Verification items for the finished model (mm, model axes). Face numbers are marked on the shaded views. A direction names the side the tool comes from. Give positions to 0.01 mm unless a question says otherwise; leave off trailing zeros. Loops run counter-clockwise (first coordinate to the right, second up) from the corner with the lowest first, then second, coordinate; pieces in that order, holes last. Notation, with made-up numbers: M 12.5,-21 L 24.5,-21 A22 ccw 24.5,-12 Z; hole C -23.75,-30 d6. An arc over 180 degrees is marked long. Use CSV: the item, a comma, the result in double quotes.
from build123d import *

# Parameters (mm, degrees)
EXTRUDE_1_DEPTH     = 29
EXTRUDE_2_DEPTH     = 5
CHAMFER_1_SIZE      = 1
SKETCH_4_W          = 2
SKETCH_4_H          = 3.10400654
SKETCH_4_H_2        = 3.326169865
CUT_EXTRUDE_1_DEPTH = 30


with BuildPart() as part:
    # 草图1 → 凸台-拉伸1 (new body)
    with BuildSketch(Plane.XY):
        Polygon((-19.832016219, -9.875726629), (-3.832016219, -9.875726629), (-8.832016219, -4.875726629), (-14.832016219, -4.875726629), align=None)
    extrude(amount=EXTRUDE_1_DEPTH)

    # 草图3 → 凸台-拉伸2 (add)
    with BuildSketch(Plane.XZ.offset(9.875726629)):
        Polygon((-11.832016219, 29), (-1.832016219, 29), (-1.832016219, 34), (-21.832016219, 34), (-21.832016219, 29), align=None)
    extrude(amount=-EXTRUDE_2_DEPTH)

    # 倒角1
    chamfer_1_edges = [part.edges().sort_by_distance(p)[0] for p in [
        (-11.832016219, -4.875726629, 0),
        (-6.332016219, -7.375726629, 0),
        (-11.832016219, -9.875726629, 0),
        (-17.332016219, -7.375726629, 0),
    ]]
    chamfer(chamfer_1_edges, length=CHAMFER_1_SIZE)

    # 草图4 → 切除-拉伸1 (cut, through all)
    with BuildSketch(Plane(origin=(0, 0, 29), x_dir=(-1, 0, 0), z_dir=(0, 0, -1))):
        with Locations((4.832016219, -8.323723359)):
            Rectangle(SKETCH_4_W, SKETCH_4_H)
        with Locations((18.832016219, -8.212641697)):
            Rectangle(SKETCH_4_W, SKETCH_4_H_2)
    extrude(amount=CUT_EXTRUDE_1_DEPTH, mode=Mode.SUBTRACT)


solid = part.part
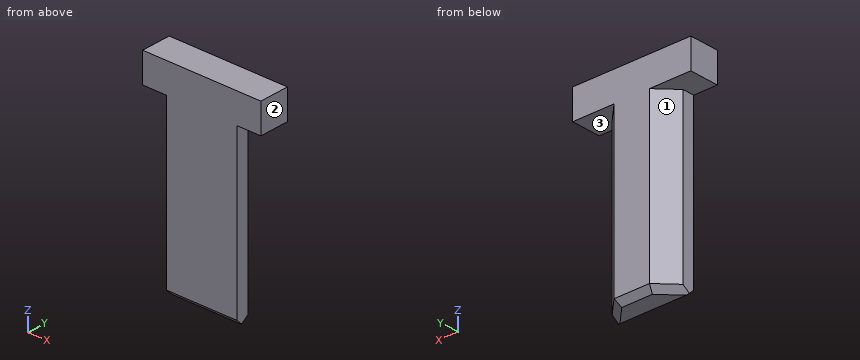
(1) Scan lines: L1, parallel to Z at x = -4.75, y = -5.1; L2, parallel to X at y = -9.5, z = 26; L3, parallel to X at y = -7.85, z = 23. Record each from-to range of solid material in increasing order. Write a range as from..to.
Calculated:
L1,"z = 29..34"
L2,"x = -17.83..-5.83"
L3,"x = -17.81..-5.86"
(2) Tool access check on the marked faces 1, 2 and 3. Record the directions out of +Z, -Z, +X, -X, +Y, -Y that give a thin tool (end or side, any length) a straight path to the whole face; none if there is none.
Calculated:
face 1,"-Z, -X, +Y"
face 2,"+Z, -Z, +X, +Y, -Y"
face 3,"-Z, +X, +Y"
(3) Section check C-C on x = -8.5. Record the cut outline in (y, z), plus the area to 3 significant figures.
Calculated:
outline,"M -9.88,1 L -8.88,0 L -6.62,0 L -5.21,1 L -5.21,29 L -4.88,29 L -4.88,34 L -9.88,34 Z"
area,"159 mm²"
(4) Depth check by flat-ended pin: pin 1 Ø2 at (y, z) = (-7.5, 7) entering from -X; pin 2 Ø2.5 at (x, y) = (-18.5, -7.5) entering from -Z; pin 3 Ø1.5 at (x, y) = (-5, -6.5) entering from -Z. Enter the tip coordinate at first touch or a pass-through.
Calculated:
pin 1,"stops at x = -17.83"
pin 2,"stops at z = 0.49"
pin 3,"stops at z = 29"
(5) Section check A-A on y = -8.35. Record the cut outline in (x, z), plus the area to 3 significant figures.
Calculated:
outline,"M -21.83,29 L -17.83,29 L -17.83,0.66 L -16.89,0 L -6.77,0 L -5.83,0.66 L -5.83,29 L -1.83,29 L -1.83,34 L -21.83,34 Z"
area,"447 mm²"
(6) Section check D-D on y = -5.3. Record the cut outline in (x, z), plus the area to 3 significant figures.
Calculated:
outline,"M -21.83,29 L -15.26,29 L -15.26,1 L -14.66,0.58 L -9.01,0.58 L -8.41,1 L -8.41,29 L -1.83,29 L -1.83,34 L -21.83,34 Z"
area,"294 mm²"
(7) Section check B-B on z = 24.5. Record the cut outline in (x, y).
Calculated:
outline,"M -17.83,-9.88 L -5.83,-9.88 L -5.83,-7.88 L -8.83,-4.88 L -14.83,-4.88 L -17.83,-7.88 Z"
